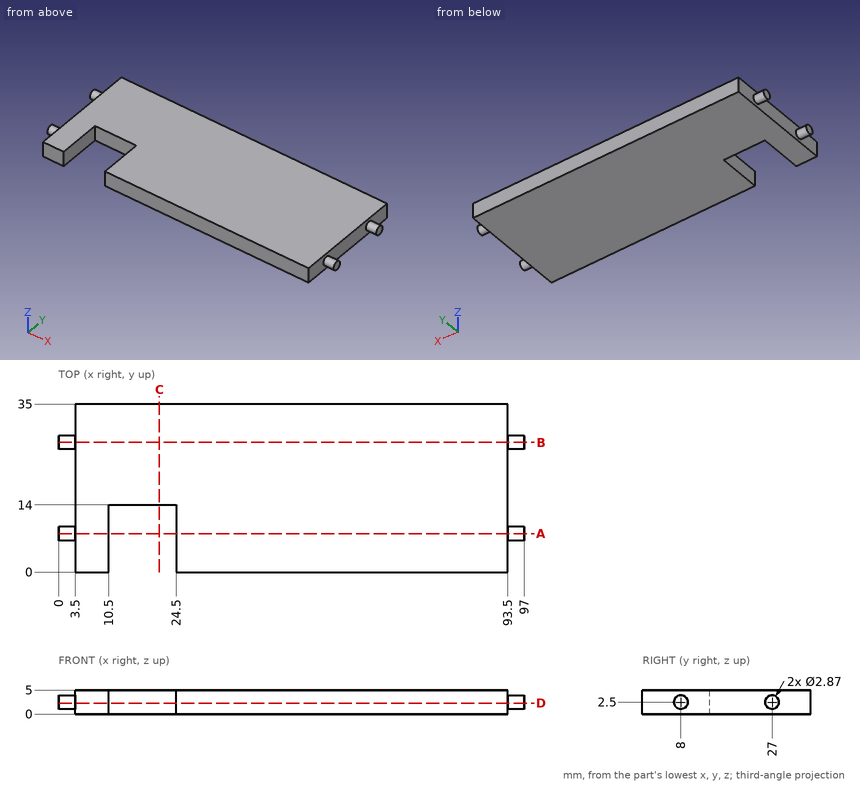
Check sheet for the drawn part. Datum: minimum x, y, z corner. Units: mm. Give positions to 0.01 mm unless a question says otherwise; leave off trailing zeros. Loops run counter-clockwise (first coordinate to the right, second up) from the corner with the lowest first, then second, coordinate; pieces in that order, holes last. Notation, with made-up numbers: (51.25, 66.25) - (99.25, 66.25) arc R34 cw to (99.25, 98.25) - close; hole circle Ø3 at (79, -29.75). An arc over 180 degrees is marked (long way). Write each question's results on one line, items separated by ' | '.
1) Sectioned sample at D-D on z = 2.3. Record the boundary of the cut face in (x, y), plus the area to 3 significant figures.
Solution:
outline: (0, 6.58) - (3.5, 6.58) - (3.5, 0) - (10.5, 0) - (10.5, 14) - (24.5, 14) - (24.5, 0) - (93.5, 0) - (93.5, 6.58) - (97, 6.58) - (97, 9.42) - (93.5, 9.42) - (93.5, 25.58) - (97, 25.58) - (97, 28.42) - (93.5, 28.42) - (93.5, 35) - (3.5, 35) - (3.5, 28.42) - (0, 28.42) - (0, 25.58) - (3.5, 25.58) - (3.5, 9.42) - (0, 9.42) - close | area: 2,990 mm2
2) Sectioned sample at A-A on y = 8. Record the boundary of the cut face in (x, z) (3 decimals).
Solution:
outline: (0, 1.065) - (3.5, 1.065) - (3.5, 0) - (10.5, 0) - (10.5, 5) - (3.5, 5) - (3.5, 3.935) - (0, 3.935) - close; (24.5, 0) - (93.5, 0) - (93.5, 1.065) - (97, 1.065) - (97, 3.935) - (93.5, 3.935) - (93.5, 5) - (24.5, 5) - close
3) Sectioned sample at C-C on x = 21. Record the boundary of the cut face in (y, z), plus the area to 3 significant figures.
Solution:
outline: (14, 0) - (35, 0) - (35, 5) - (14, 5) - close | area: 105 mm2
4) Sectioned sample at B-B on y = 27. Record the boundary of the cut face in (x, z) (3 decimals).
Solution:
outline: (0, 1.065) - (3.5, 1.065) - (3.5, 0) - (93.5, 0) - (93.5, 1.065) - (97, 1.065) - (97, 3.935) - (93.5, 3.935) - (93.5, 5) - (3.5, 5) - (3.5, 3.935) - (0, 3.935) - close
5) Depth check by flat-ended pin: P1, Ø8, axis at x = 19.5, y = 20, coming from the -Z side; P2, Ø3, axis at y = 30.5, z = 3.5, coming from the +X side. Enter the tip coordinate at first touch or a pass-through.
Solution:
P1: z = 0 | P2: x = 93.5
6) Material ranges on L1, parallel to X at y = 3, z = 0.75; L2, parallel to X at y = 20.5, z = 4.65; L3, parallel to Y at x = 17.5, z = 2.65, recorded low to high. Write a range as from..to.
Solution:
L1: 3.5..10.5, 24.5..93.5 | L2: 3.5..93.5 | L3: 14..35
